Geometry check sheet. Reference: the model listing, model coordinates, mm. Give positions to 0.01 mm unless a question says otherwise; leave off trailing zeros. Order: outer loops, then holes, each group sorted by start corner. A loop starts at its lowest first (then second) coordinate and runs counter-clockwise, first axis right, second up.
from build123d import *

# Parameters (mm, degrees)
F0_W     = 101.5
F0_H     = 15.875
F0_W_2   = 72.5
F0_H_2   = 3
F0_W_3   = 66.5
F0_R     = 1.5
F1_DEPTH = 3.5
F2_W     = 78.5
F2_H     = 15.875
F3_DEPTH = 0.5
F4_R     = 2.5
F5_DEPTH = 25


with BuildPart() as f1:
    # F0 (on Front) → F1 (new body)
    with BuildSketch(Plane.XZ):
        Rectangle(F0_W, F0_H)
        with Locations((0, -2.5625)):
            Rectangle(F0_W_2, F0_H_2, mode=Mode.SUBTRACT)
        with Locations((-3, 3.4375)):
            Rectangle(F0_W_3, F0_H_2, mode=Mode.SUBTRACT)
        with Locations((34.75, 3.4375)):
            Circle(F0_R, mode=Mode.SUBTRACT)
    extrude(amount=F1_DEPTH)

    # F2 (on face) → F3 (cut)
    with BuildSketch(Plane(origin=(0, 0, 0), x_dir=(-1, 0, 0), z_dir=(0, 1, 0))):
        Rectangle(F2_W, F2_H)
    extrude(amount=-F3_DEPTH, mode=Mode.SUBTRACT)

    # F4 (on face) → F5 (cut)
    with BuildSketch(Plane.XZ.offset(3.5)):
        with Locations((-45, 0)):
            Circle(F4_R)
        with Locations((45, 0)):
            Circle(F4_R)
    extrude(amount=-F5_DEPTH, mode=Mode.SUBTRACT)


solid = f1.part
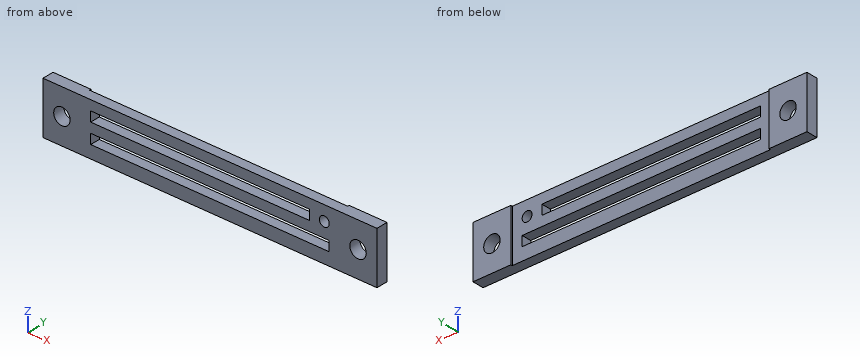
Item 1: Sectioned sample at B-B (z = 0). Enter the section's corners in (x, y), and give its area (3 significant figures).
Reported:
outline: (-50.75, -3.5) - (-47.5, -3.5) - (-47.5, 0) - (-50.75, 0) - close; (-42.5, -3.5) - (42.5, -3.5) - (42.5, 0) - (39.25, 0) - (39.25, -0.5) - (-39.25, -0.5) - (-39.25, 0) - (-42.5, 0) - close; (47.5, -3.5) - (50.75, -3.5) - (50.75, 0) - (47.5, 0) - close
area: 281 mm2
Item 2: Sectioned sample at C-C (x = 45). Enter the section's corners in (y, z), and give its area (3 significant figures).
Reported:
outline: (-3.5, -7.94) - (0, -7.94) - (0, -2.5) - (-3.5, -2.5) - close; (-3.5, 2.5) - (0, 2.5) - (0, 7.94) - (-3.5, 7.94) - close
area: 38.1 mm2
Item 3: Scan lines: L1, parallel to Z at x = 3.5, y = -3.1; L2, parallel to Z at x = 45, y = -1.05; L3, parallel to X at y = -1.4, z = -1.25. Record each from-to range of solid material in increasing order.
Reported:
L1: z = -7.94 to -4.06, -1.06 to 1.94, 4.94 to 7.94
L2: z = -7.94 to -2.5, 2.5 to 7.94
L3: x = -50.75 to -47.17, -42.83 to -36.25, 36.25 to 42.83, 47.17 to 50.75
Item 4: Sectioned sample at D-D (y = -2.1). Enter the section's corners in (x, z), and give its area (3 significant figures).
Reported:
outline: (-50.75, -7.94) - (50.75, -7.94) - (50.75, 7.94) - (-50.75, 7.94) - close; hole circle Ø5 at (-45, 0); hole (-36.25, -4.06) - (36.25, -4.06) - (36.25, -1.06) - (-36.25, -1.06) - close; hole (-36.25, 1.94) - (30.25, 1.94) - (30.25, 4.94) - (-36.25, 4.94) - close; hole circle Ø3 at (34.75, 3.44); hole circle Ø5 at (45, 0)
area: 1,150 mm2
Item 5: Sectioned sample at A-A (x = 28). Enter the section's corners in (y, z), and give its area (3 significant figures).
Reported:
outline: (-3.5, -7.94) - (-0.5, -7.94) - (-0.5, -4.06) - (-3.5, -4.06) - close; (-3.5, -1.06) - (-0.5, -1.06) - (-0.5, 1.94) - (-3.5, 1.94) - close; (-3.5, 4.94) - (-0.5, 4.94) - (-0.5, 7.94) - (-3.5, 7.94) - close
area: 29.6 mm2
Item 6: Gauge pin test, flat ends, axial feed: pin 1 (2.5 mm diameter, centred on x = 34.75, z = 3.44, fed in from -Y); pin 2 (8 mm diameter, centred on x = -13.5, z = 1.5, fed in from +Y). Record the tip position at first contact, or that the pin passes through.
Reported:
pin 1: passes through
pin 2: stops at y = -0.5
